from build123d import *

# Parameters (mm, degrees)
SKETCH1_W           = 59.5
SKETCH1_H           = 50
SKETCH1_R           = 3
BOSS_EXTRUDE1_DEPTH = 1.5
BOSS_EXTRUDE2_DEPTH = 50
CUT_EXTRUDE1_DEPTH  = 2
CHAMFER1_SIZE       = 2
SKETCH4_W           = 59.5
SKETCH4_H           = 1.892701509
CUT_EXTRUDE2_DEPTH  = 59.318629099


with BuildPart() as part:
    # Sketch1 → Boss-Extrude1 (new body)
    with BuildSketch(Plane(origin=(0, 0, 0), x_dir=(1, 0, 0), z_dir=(0, 1, 0))):
        Rectangle(SKETCH1_W, SKETCH1_H)
        with Locations(Location((0, 0, 0), (0, 0, 270))):
            Circle(SKETCH1_R, mode=Mode.SUBTRACT)
    extrude(amount=BOSS_EXTRUDE1_DEPTH)

    # Sketch2 → Boss-Extrude2 (add)
    with BuildSketch(Plane(origin=(0, 0, -25), x_dir=(-1, 0, 0), z_dir=(0, 0, -1))):
        Polygon((-29.75, 1.5), (29.75, 1.5), (29.75, 2.5), (28.56, 4), (27.37, 2.5), (26.18, 4), (24.99, 2.5), (23.8, 4), (22.61, 2.5), (21.42, 4), (20.23, 2.5), (19.04, 4), (17.85, 2.5), (16.66, 4), (15.47, 2.5), (14.28, 4), (13.09, 2.5), (11.9, 4), (10.71, 2.5), (9.52, 4), (8.33, 2.5), (7.14, 4), (5.95, 2.5), (4.76, 4), (3.57, 2.5), (2.38, 4), (1.19, 2.5), (0, 4), (-1.19, 2.5), (-2.38, 4), (-3.57, 2.5), (-4.76, 4), (-5.95, 2.5), (-7.14, 4), (-8.33, 2.5), (-9.52, 4), (-10.71, 2.5), (-11.9, 4), (-13.09, 2.5), (-14.28, 4), (-15.47, 2.5), (-16.66, 4), (-17.85, 2.5), (-19.04, 4), (-20.23, 2.5), (-21.42, 4), (-22.61, 2.5), (-23.8, 4), (-24.99, 2.5), (-26.18, 4), (-27.37, 2.5), (-28.56, 4), (-29.75, 2.5), align=None)
    extrude(amount=-BOSS_EXTRUDE2_DEPTH)

    # Sketch3 → Cut-Extrude1 (cut)
    with BuildSketch(Plane(origin=(0, 0, 0), x_dir=(-1, 0, 0), z_dir=(0, -1, 0))):
        with BuildLine():
            Line((-1.75, -2.436698586), (-1.75, -5))
            Line((-1.75, -5), (1.75, -5))
            Line((1.75, -5), (1.75, -2.436698586))
            ThreePointArc((1.75, -2.436698586), (0, 3), (-1.75, -2.436698586))
        make_face()
    extrude(amount=-CUT_EXTRUDE1_DEPTH, mode=Mode.SUBTRACT)

    # Chamfer1
    chamfer1_edges = [part.edges().sort_by_distance(p)[0] for p in [
        (0, 0, 5),
    ]]
    chamfer(chamfer1_edges, length=CHAMFER1_SIZE - 0.0001)  # a hair under: the kernel refuses the full size

    # Sketch4 → Cut-Extrude2 (cut, through all)
    with BuildSketch(Plane.XY.offset(25)):
        with Locations((0, 3.446350755)):
            Rectangle(SKETCH4_W, SKETCH4_H)
    extrude(amount=-CUT_EXTRUDE2_DEPTH, mode=Mode.SUBTRACT)


solid = part.part
Design review of the part built by this model. Coordinates are the model's own, in mm. A direction names the side the tool comes from. Coordinates: 2 decimals unless noted, no trailing zeros. Write each loop counter-clockwise with the first axis right and the second up, starting at its lowest first coordinate (ties: lowest second). Pieces come first, ordered by that corner, then holes. Notation, with made-up numbers: (22, -21.5) - (49, -21.5) arc R18 ccw to (49, -5.5) - close; hole circle Ø2 at (11, 29.25). An arc over 180 degrees is marked (long way). One line per item, written item: value.
1) Mouldability with a two-part tool opening along Z and no side actions: class faces 3 (the face through (-1.75, 1, 4)), 4 (the face through (0, 1, -25)), 5 (the face through (-29.75, 1, 0)) as +Z half, -Z half, draft (parallel to the pull), parting line (faces both ways), or undercut.
Answer sheet:
face 3: undercut
face 4: -Z half
face 5: draft
2) Add section B-B (z = 0). State the section outline as (x, y) points, plus the area to 3 significant figures.
Answer sheet:
outline: (-29.75, 0) - (-3, 0) - (-3, 2) - (3, 2) - (3, 0) - (29.75, 0) - (29.75, 2.5) - (-29.75, 2.5) - close
area: 137 mm2
3) To check wall thickness, follow probe 1 along X at (y, z) = (0.25, 4); probe 2 along X at (y, z) = (1.7, 0); probe 3 along Z at (x, y) = (0, 1.6). State the ranges of each line that lie inside material, in increasing order.
Answer sheet:
probe 1: x = -29.75 to -1.75, 1.75 to 29.75
probe 2: x = -29.75 to -3, 3 to 29.75
probe 3: z = -25 to -3, 5.4 to 25
4) Insertion check: pin 1 (3 mm diameter, centred on x = 1, z = 0.5, fed in from -Y). The pin has a flat end and moves straight along its axis. Give the tip position at first contact, or say it passes through.
Answer sheet:
pin 1: stops at y = 2
5) For faces 1 (the face through (0, 0, -6)), 2 (the face through (1.75, 1, 4)), list the 3-axis set-ups (+Z, -Z, +X, -X, +Y, -Y) from which the entire face can be reached by the end or side of a thin tool; tool diameter is ignored.
Answer sheet:
face 1: +Z, -Z, +X, -X, -Y
face 2: -Y
